Here's the drawing with two shaded views (mm, measured from the low corner). I have some questions. Coordinates: 2 decimals unless noted, no trailing zeros. Answer as a JSON object with one key per item and string values. Group by question number.
Q1. I'm going to push flat-ended pins straight in: pin 1 (5 mm diameter, centred on y = 114.5, z = 3.5, fed in from +X) (3 decimals); pin 2 (7.5 mm diameter, centred on x = 15.5, y = 225, fed in from -Z) (3 decimals); pin 3 (5 mm diameter, centred on x = 16, y = 101, fed in from +Z) (3 decimals). Where does each tip first touch, or does it pass through?
Q2. I want a section at A-A on y = 44.45. Count the separate pieces of the cut face and the enclosed holes in it, then the cut area to 3 significant figures.
Q3. I need wall thicknesses on line 1 (Z direction, x = 4, y = 44.45); line 2 (Z direction, x = 18, y = 268) (1 decimal); line 3 (Y direction, x = 7.25, z = 283) (1 decimal). Which ranges of each line are inside material? Lowest first, please.
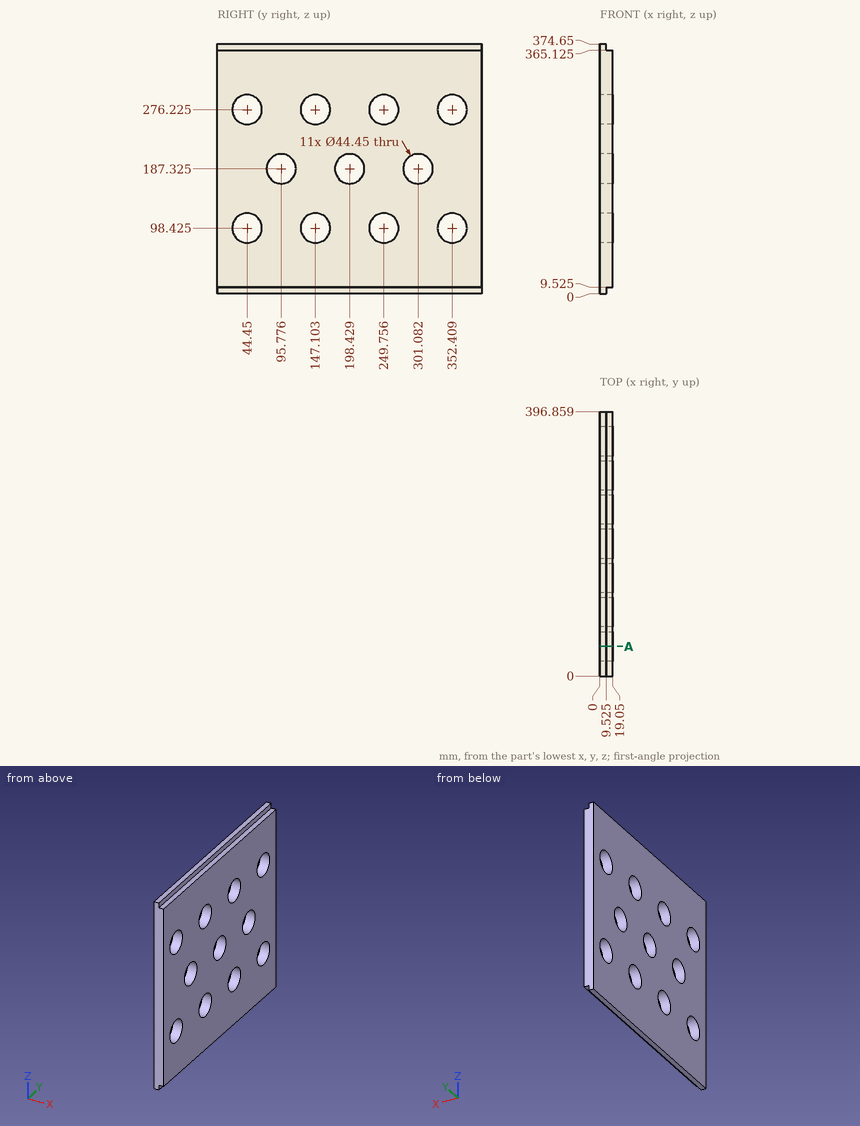
Result set:
{
 "1": {"pin 1": "stops at x = 9.525", "pin 2": "stops at z = 9.525", "pin 3": "stops at z = 365.125"},
 "2": {"separate pieces": "3", "enclosed holes": "0", "area": "5,260 mm²"},
 "3": {"line 1": "z = 0 to 76.2, 120.65 to 254, 298.45 to 374.65", "line 2": "z = 9.5 to 85.7, 111.1 to 263.5, 288.9 to 365.1", "line 3": "y = 0 to 23.3, 65.6 to 125.9, 168.3 to 228.6, 270.9 to 331.2, 373.6 to 396.9"}
}
